Build history of the part. All positions in model axes, mm. Give positions to 0.01 mm unless a question says otherwise; leave off trailing zeros. Write each loop counter-clockwise with the first axis right and the second up, starting at its lowest first coordinate (ties: lowest second). Pieces come first, ordered by that corner, then holes. Notation, with made-up numbers: (10.25, 1) -> (65.25, 1) arc R27 cw to (65.25, 31) -> close; hole circle Ø11 at (-32, 65.25). An arc over 180 degrees is marked (long way). Put each result on its own line as item: value.
from build123d import *

# Parameters (mm, degrees)
F0_W     = 50.8
F0_H     = 25.4
F0_W_2   = 47.625
F0_H_2   = 22.225
F1_DEPTH = 304.8
F3_D     = 5.1054
F5_D     = 5.1054


with BuildPart() as f1:
    # F0 (on Right) → F1 (new body)
    with BuildSketch(Plane.YZ):
        Rectangle(F0_W, F0_H)
        Rectangle(F0_W_2, F0_H_2, mode=Mode.SUBTRACT)
    extrude(amount=F1_DEPTH)

    # F3 (through all)
    with Locations(Plane.XY.offset(12.7)):
        with Locations((38.1, -12.7), (63.5, 12.7), (63.5, -12.7), (88.9, 12.7), (88.9, -12.7), (114.3, 12.7), (292.1, -12.7), (266.7, -12.7), (241.3, -12.7), (215.9, -12.7), (190.5, -12.7), (165.1, -12.7), (292.1, 12.7), (266.7, 12.7), (241.3, 12.7), (215.9, 12.7), (114.3, -12.7), (190.5, 12.7), (139.7, 12.7), (139.7, -12.7), (165.1, 12.7), (12.7, 12.7), (12.7, -12.7), (38.1, 12.7)):
            Hole(F3_D / 2)

    # F5 (through all)
    with Locations(Plane(origin=(0, 25.4, 0), x_dir=(-1, 0, 0), z_dir=(0, 1, 0))):
        with Locations((-215.9, 0), (-241.3, 0), (-190.5, 0), (-139.7, 0), (-165.1, 0), (-88.9, 0), (-114.3, 0), (-266.7, 0), (-292.1, 0), (-12.7, 0), (-38.1, 0), (-63.5, 0)):
            Hole(F5_D / 2)


solid = f1.part
1) Pull direction X, two halves, no side cores. Call faces 1 (the flat face through (0, 0, -12)), 2 (the flat face through (150, 23.812, 0)), 3 (the cylindrical face through (238.865, 13.467, 11.895)): released by +X, released by -X, zero draft, split by the parting line, or undercut.
Filled sheet:
face 1: released by -X
face 2: zero draft
face 3: undercut
2) Slice it at A-A (z = 8.5). Write the cut outline in (x, y), plus the area to 3 significant figures.
Filled sheet:
outline: (0, -25.4) -> (304.8, -25.4) -> (304.8, -23.81) -> (0, -23.81) -> close; (0, 23.81) -> (304.8, 23.81) -> (304.8, 25.4) -> (0, 25.4) -> close
area: 968 mm2
3) Wall check: L1, parallel to Y at x = 88.9, z = 11.7; L2, parallel to Z at x = 176, y = 11.5; L3, parallel to Y at x = 99.5, z = -4. Give the ranges that are in metal, low to high.
Filled sheet:
L1: -25.4 to -15.25, -10.15 to 10.15, 15.25 to 25.4
L2: -12.7 to -11.11, 11.11 to 12.7
L3: -25.4 to -23.81, 23.81 to 25.4
4) Slice it at B-B (y = 20.5). Write the cut outline in (x, z), plus the area to 3 significant figures.
Filled sheet:
outline: (0, -12.7) -> (304.8, -12.7) -> (304.8, -11.11) -> (0, -11.11) -> close; (0, 11.11) -> (304.8, 11.11) -> (304.8, 12.7) -> (0, 12.7) -> close
area: 968 mm2
5) Slice it at C-C (x = 69). Write the cut outline in (y, z), plus the area to 3 significant figures.
Filled sheet:
outline: (-25.4, -12.7) -> (25.4, -12.7) -> (25.4, 12.7) -> (-25.4, 12.7) -> close; hole (-23.81, -11.11) -> (23.81, -11.11) -> (23.81, 11.11) -> (-23.81, 11.11) -> close
area: 232 mm2
